Geometry: see drawing. Coordinates: mm, zero at the bounding-box minimum. Coordinates: 2 decimals unless noted, no trailing zeros. Write each loop counter-clockwise with the first axis right and the second up, starting at its lowest first coordinate (ties: lowest second). Pieces come first, ordered by that corner, then holes. Notation, with made-up numbers: M 3.5,-17 L 41.5,-17 A37 ccw 41.5,20 Z; hole C -23,61.5 d6. An arc over 180 degrees is marked long. Answer as CSV lines item,"result". Start each with the question number.
1. Contact query for flat-ended pins moving along their axis: pin 1 Ø3 at (x, z) = (11, 24) entering from -Y (1 decimal); pin 2 Ø1.5 at (y, z) = (13.5, 77.5) entering from -X; pin 3 Ø3 at (y, z) = (17.5, 49.5) entering from -X; pin 4 Ø13 at (x, y) = (26.67, 26.67) entering from -Z. Output: stop coordinate, or through.
2. Line query: probe 1 along Y at (x, z) = (26.67, 33); probe 2 along Y at (x, z) = (26, 53); probe 3 along Z at (x, y) = (19.5, 36) (1 decimal). Output: solid intervals per line, ascending. Write a range as [from, to].
3. Section A-A on y = 26.67. Return the cut outline in (x, z), plus the area to 3 significant figures.
4. Section C-C on z = 60. Return the cut outline in (x, y).
5. Section D-D on z = 116. Return the cut outline in (x, y), plus the area to 3 significant figures.
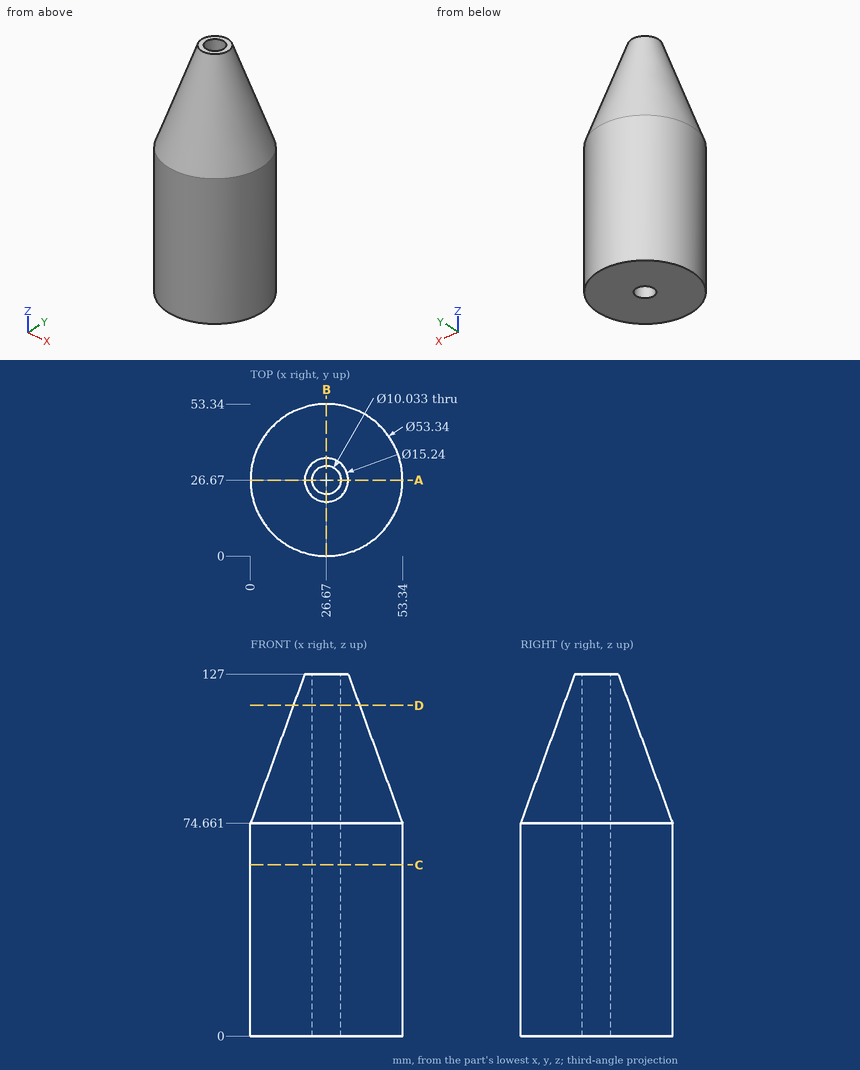
Values:
1,pin 1,"y = 4.1"
1,pin 2,"x = 4.14"
1,pin 3,"x = 1.13"
1,pin 4,"z = 0"
2,probe 1,"[0, 21.65], [31.69, 53.34]"
2,probe 2,"[0.01, 21.7], [31.64, 53.33]"
2,probe 3,"[0, 115.6]"
3,outline,"M 0,0 L 21.65,0 L 21.65,127 L 19.05,127 L 0,74.66 Z; M 31.69,0 L 53.34,0 L 53.34,74.66 L 34.29,127 L 31.69,127 Z"
3,area,"4,500 mm²"
4,outline,"C 26.67,26.67 d53.34; hole C 26.67,26.67 d10.03"
5,outline,"C 26.67,26.67 d23.25; hole C 26.67,26.67 d10.03"
5,area,"345 mm²"
